from build123d import *

# Parameters (mm, degrees)
EXTRUDE_1_DEPTH     = 73
SKETCH_2_W          = 32
SKETCH_2_H          = 17
EXTRUDE_2_DEPTH     = 10
SKETCH_3_W          = 6
SKETCH_3_H          = 22
CUT_EXTRUDE_1_DEPTH = 95.605760924
SKETCH_4_R          = 2.25
CUT_EXTRUDE_2_DEPTH = 10


with BuildPart() as part:
    # 草图1 → 凸台-拉伸1 (new body)
    with BuildSketch(Plane(origin=(0, 0, 0), x_dir=(1, 0, 0), z_dir=(0, 1, 0))):
        Polygon((-36.5, 30), (36.5, 30), (30, 0), (-30, 0), align=None)
    extrude(amount=EXTRUDE_1_DEPTH)

    # 草图2 → 凸台-拉伸2 (add)
    with BuildSketch(Plane(origin=(0, 73, 0), x_dir=(1, 0, 0), z_dir=(0, 1, 0))):
        with Locations((0, 21.5)):
            Rectangle(SKETCH_2_W, SKETCH_2_H)
    extrude(amount=EXTRUDE_2_DEPTH)

    # 草图3 → 切除-拉伸1 (cut, through all)
    with BuildSketch(Plane(origin=(0, 0, -27), x_dir=(-1, 0, 0), z_dir=(0, 0, -1))):
        with Locations((-33.5, 36.5)):
            Rectangle(SKETCH_3_W, SKETCH_3_H)
        with Locations((33.5, 36.5)):
            Rectangle(SKETCH_3_W, SKETCH_3_H)
    extrude(amount=-CUT_EXTRUDE_1_DEPTH, mode=Mode.SUBTRACT)

    # 草图4 → 切除-拉伸2 (cut)
    with BuildSketch(Plane.XY.offset(-27)):
        with Locations((32.85, 36.5)):
            Circle(SKETCH_4_R)
        with Locations((-32.85, 36.5)):
            Circle(SKETCH_4_R)
    extrude(amount=-CUT_EXTRUDE_2_DEPTH, mode=Mode.SUBTRACT)


solid = part.part
Read the model definition and answer for the solid it produces. Units are mm, in the model's axes. A direction names the side the tool comes from. Round coordinates to 2 decimals unless told otherwise and drop trailing zeros. Write each loop counter-clockwise with the first axis right and the second up, starting at its lowest first coordinate (ties: lowest second). Pieces come first, ordered by that corner, then holes.
Q1. Find section A-A on y = 28. Determine the outline of the cut face in (x, z), and give its area (3 significant figures).
Values:
outline: (-36.5, -30) - (36.5, -30) - (35.85, -27) - (30.5, -27) - (30.5, -2.31) - (30, 0) - (-30, 0) - (-30.5, -2.31) - (-30.5, -27) - (-35.85, -27) - close
area: 1,860 mm2
Q2. Find section D-D on z = -18.75. Determine the outline of the cut face in (x, y), and give its area (3 significant figures).
Values:
outline: (-34.06, 0) - (34.06, 0) - (34.06, 25.5) - (30.5, 25.5) - (30.5, 47.5) - (34.06, 47.5) - (34.06, 73) - (16, 73) - (16, 83) - (-16, 83) - (-16, 73) - (-34.06, 73) - (-34.06, 47.5) - (-30.5, 47.5) - (-30.5, 25.5) - (-34.06, 25.5) - close
area: 5,140 mm2
Q3. Find section B-B on x = -5. Determine the outline of the cut face in (y, z).
Values:
outline: (0, -30) - (83, -30) - (83, -13) - (73, -13) - (73, 0) - (0, 0) - close
Q4. A tool of negligible diameter and unlimited length cuts with its end or side. For faces 5 (the face through (0, 78, -13)), 6 (the face through (-33, 25.5, -18)), 7 (the face through (32, 25.5, -20)), 8 (the face through (16, 78, -21)), 9 (the face through (-16, 78, -21)), from which of +Z, -Z, +X, -X, +Y, -Y can it reach the whole face along a straight path? Write none if from no direction.
Values:
face 5: +Z, +X, -X, +Y
face 6: +Z, -X
face 7: +Z, +X
face 8: +Z, -Z, +X, +Y
face 9: +Z, -Z, -X, +Y
Q5. The mould has two halves that part along X. Classify faces 1 (the face through (-30.316, 35.989, -1.457)), 2 (the face through (30.5, 36, -15)), 3 (the face through (-31.64, 38.397, -28.479)), 4 (the face through (0, 83, -22)): released by +X, released by -X, zero draft, split by the parting line, or undercut.
Values:
face 1: released by -X
face 2: released by +X
face 3: undercut
face 4: zero draft
Q6. Straight lines are drawn through the part: line 1 (Y direction, x = 32.85, z = -28.2); line 2 (X direction, y = 47, z = -24.5); line 3 (X direction, y = 76, z = -27.75). For each, find the intervals that lie inside material, in ascending order.
Values:
line 1: y = 0 to 34.25, 38.75 to 73
line 2: x = -30.5 to 30.5
line 3: x = -16 to 16
Q7. Find section C-C on x = -32.85. Determine the outline of the cut face in (y, z).
Values:
outline: (0, -30) - (34.25, -30) - (34.25, -27) - (25.5, -27) - (25.5, -13.15) - (0, -13.15) - close; (38.75, -30) - (73, -30) - (73, -13.15) - (47.5, -13.15) - (47.5, -27) - (38.75, -27) - close
Q8. Flat-ended cylindrical pins translate along their axes: P1, Ø4.5, axis at x = -33.5, z = -13.5, coming from the +Y side; P2, Ø8, axis at y = 75.5, z = -20, coming from the -X side; P3, Ø8, axis at x = 6, y = 79, coming from the +Z side; P4, Ø4, axis at x = 32.85, y = 36.5, coming from the +Z side. Find the tip coordinate at first contact, or state that the pin passes through.
Values:
P1: stops at y = 73
P2: stops at x = -35.01
P3: stops at z = -13
P4: passes through
